Check sheet for the modelled part. Datum: model origin and axes. Units: mm. A direction names the side the tool comes from. Round coordinates to 2 decimals unless told otherwise and drop trailing zeros. Loops run counter-clockwise (first coordinate to the right, second up) from the corner with the lowest first, then second, coordinate; pieces in that order, holes last. Notation, with made-up numbers: (27, 47) -> (79, 47) arc R23 cw to (79, 85) -> close; hole circle Ø6 at (45.5, 75). An arc over 180 degrees is marked (long way). Use one line per item in the form item = value. Start each with the question number.
(1) Set-up check for faces 4 (the flat face through (0.86, 1.16, 0.51)), 5 (the flat face through (0, -20, 0)), 6 (the cylindrical face through (1, -10, 0)): record each of +Z, -Z, +X, -X, +Y, -Y from which the full face is reachable in a straight line by a thin tool's end or side.
(2) Sectioned sample at B-B (y = -8). Record the cut outline in (x, z), and give its area (3 significant figures).
(3) Go/stop test with flat-tipped pins: pin 1 (1.5 mm diameter, centred on x = -0.5, y = -1, fed in from -Z); pin 2 (1 mm diameter, centred on x = 0, y = -3, fed in from +Z). Record where each tip stops, or that it passes through.
(4) Sectioned sample at A-A (x = 0). Record the cut outline in (y, z), and give its area (3 significant figures).
(5) Material ranges on probe 1 along Y at (x, z) = (0.3, 1.55); probe 2 along Y at (x, z) = (0.55, -0.2); probe 3 along Z at (x, y) = (0.7, 0.75), recorded low to high. Write a range as [from, to].
(6) Draft check along X on faces 1 (the flat face through (-1, 0, 1)), 2 (the cylindrical face through (-2, 1, 0)), 3 (the flat face through (0, 1, 1)). Enter one of: released by +X, released by -X, zero draft, split by the parting line, or undercut.
from build123d import *

# Parameters (mm, degrees)
SKETCH1_R           = 2
BOSS_EXTRUDE1_DEPTH = 2
CHAMFER1_SIZE       = 0.3
CUT_EXTRUDE1_DEPTH  = 1.5
CHAMFER2_SIZE       = 0.2
SKETCH3_R           = 1
BOSS_EXTRUDE2_DEPTH = 20
CHAMFER3_SIZE       = 0.2


with BuildPart() as part:
    # Sketch1 → Boss-Extrude1 (new body)
    with BuildSketch(Plane(origin=(0, 0, 0), x_dir=(1, 0, 0), z_dir=(0, 1, 0))):
        with Locations(Location((0, 0, 0), (0, 0, 270))):  # turned: the seam where the file's is
            Circle(SKETCH1_R)
    extrude(amount=BOSS_EXTRUDE1_DEPTH)

    # Chamfer1
    chamfer1_edges = [part.edges().sort_by_distance(p)[0] for p in [
        (0, 2, -2),
    ]]
    chamfer(chamfer1_edges, length=CHAMFER1_SIZE)

    # Sketch2 → Cut-Extrude1 (cut)
    with BuildSketch(Plane(origin=(0, 2, 0), x_dir=(1, 0, 0), z_dir=(0, 1, 0))):
        Polygon((1.154700538, 0), (0.577350269, 1), (-0.577350269, 1), (-1.154700538, 0), (-0.577350269, -1), (0.577350269, -1), align=None)
    extrude(amount=-CUT_EXTRUDE1_DEPTH, mode=Mode.SUBTRACT)

    # Chamfer2
    chamfer2_edges = [part.edges().sort_by_distance(p)[0] for p in [
        (0.866025404, 2, 0.5),
        (0.866025404, 2, -0.5),
        (0, 2, -1),
        (-0.866025404, 2, -0.5),
        (-0.866025404, 2, 0.5),
        (0, 2, 1),
    ]]
    chamfer(chamfer2_edges, length=CHAMFER2_SIZE)

    # Sketch3 → Boss-Extrude2 (add)
    with BuildSketch(Plane.XZ):
        with Locations(Location((0, 0, 0), (0, 0, 90))):  # turned: the seam where the file's is
            Circle(SKETCH3_R)
    extrude(amount=BOSS_EXTRUDE2_DEPTH)

    # Chamfer3
    chamfer3_edges = [part.edges().sort_by_distance(p)[0] for p in [
        (0, -20, -1),
    ]]
    chamfer(chamfer3_edges, length=CHAMFER3_SIZE)


solid = part.part
Checks:
q1.face_4 = +Y
q1.face_5 = +Z, -Z, +X, -X, -Y
q1.face_6 = -Y
q2.outline = circle Ø2 at (0, 0)
q2.area = 3.14 mm2
q3.pin_1 = -1
q3.pin_2 = 1
q4.outline = (-20, -0.8) -> (-19.8, -1) -> (0, -1) -> (0, -2) -> (1.7, -2) -> (2, -1.7) -> (2, -1.2) -> (1.8, -1) -> (0.5, -1) -> (0.5, 1) -> (1.8, 1) -> (2, 1.2) -> (2, 1.7) -> (1.7, 2) -> (0, 2) -> (0, 1) -> (-19.8, 1) -> (-20, 0.8) -> close
q4.area = 44.8 mm2
q5.probe_1 = [0, 2]
q5.probe_2 = [-20, 0.5]
q5.probe_3 = [-1.87, -0.79], [0.79, 1.87]
q6.face_1 = zero draft
q6.face_2 = split by the parting line
q6.face_3 = undercut
